```python
from build123d import *

# Parameters (mm, degrees)
F0_R        = 10
F1_DEPTH    = 25
F2_DEPTH    = 25
F3_T2_ANGLE = 203.6133668192
F3_T8_ANGLE = 184.7022290241


# Not quite as in the source:
# - a fillet or chamfer that OpenCascade refuses, or shapes differently, is made with other operations: its cross-section is extruded or revolved along the edge and cut away or added


with BuildPart() as f1:
    # F0 (on Front) → F1 (new body)
    with BuildSketch(Plane.XZ):
        with BuildLine():
            Line((4.1054428346, 24.6606029758), (0, 25))
            ThreePointArc((0, 25), (-25, 0), (0, -25))
            Line((0, -25), (4.1054428346, -24.6606029758))
            ThreePointArc((4.1054428346, -24.6606029758), (19.0740146648, -16.1611251022), (25, 0))
            ThreePointArc((25, 0), (19.0740146648, 16.1611251022), (4.1054428346, 24.6606029758))
        make_face()
        Circle(F0_R, mode=Mode.SUBTRACT)
        with BuildLine():
            ThreePointArc((4.1054428346, 24.6606029758), (2.0597239626, 24.9150062653), (0, 25))
            Line((0, 25), (4.1054428346, 24.6606029758))
        make_face()
        with BuildLine():
            Line((4.1054428346, -24.6606029758), (0, -25))
            ThreePointArc((0, -25), (2.0597239626, -24.9150062653), (4.1054428346, -24.6606029758))
        make_face()
        with BuildLine():
            Line((91.4418067738, 17.4405043857), (4.1054428346, 24.6606029758))
            ThreePointArc((4.1054428346, 24.6606029758), (19.0740146648, 16.1611251022), (25, 0))
            ThreePointArc((25, 0), (19.0740146648, -16.1611251022), (4.1054428346, -24.6606029758))
            Line((4.1054428346, -24.6606029758), (91.4418067738, -17.4405043857))
            ThreePointArc((91.4418067738, -17.4405043857), (72.5, 0), (91.4418067738, 17.4405043857))
        make_face()
        with BuildLine():
            ThreePointArc((107.5, 0), (102.8740362463, 11.8536572723), (91.4418067738, 17.4405043857))
            ThreePointArc((91.4418067738, 17.4405043857), (72.5, 0), (91.4418067738, -17.4405043857))
            ThreePointArc((91.4418067738, -17.4405043857), (102.8740362463, -11.8536572723), (107.5, 0))
        make_face()
        with Locations((90, 0)):
            Circle(F0_R, mode=Mode.SUBTRACT)
    extrude(amount=-F1_DEPTH)

    # F0 (on Front) → F2 (join)
    with BuildSketch(Plane.XZ):
        with BuildLine():
            Line((4.1054428346, 24.6606029758), (0, 25))
            ThreePointArc((0, 25), (-25, 0), (0, -25))
            Line((0, -25), (4.1054428346, -24.6606029758))
            ThreePointArc((4.1054428346, -24.6606029758), (19.0740146648, -16.1611251022), (25, 0))
            ThreePointArc((25, 0), (19.0740146648, 16.1611251022), (4.1054428346, 24.6606029758))
        make_face()
        Circle(F0_R, mode=Mode.SUBTRACT)
    extrude(amount=F2_DEPTH)

    # F3: chamfer of 2 on 4 edges, made by hand

    # F3_s1 → F3_t2 (revolve, cut)
    with BuildSketch(Plane(origin=(0, 0, 0), x_dir=(0, 1, 0), z_dir=(0.9788435281, 0, -0.2046102329))):
        Polygon((-23, 25), (-25, 23), (-25, 25), align=None)
    revolve(axis=Axis((0, -25, 0), (0, -1, 0)), revolution_arc=F3_T2_ANGLE, mode=Mode.SUBTRACT)

    # F3_s3 → F3_t4 (revolve, cut)
    with BuildSketch(Plane.XY):
        Polygon((102, 0), (100, 2), (100, 0), align=None)
    revolve(axis=Axis((90, 0, 0), (0, -1, 0)), mode=Mode.SUBTRACT)

    # F3_s5 → F3_t6 (revolve, cut)
    with BuildSketch(Plane.XY):
        Polygon((12, -25), (10, -23), (10, -25), align=None)
    revolve(axis=Axis((0, -25, 0), (0, -1, 0)), mode=Mode.SUBTRACT)

    # F3_s7 → F3_t8 (revolve, cut)
    with BuildSketch(Plane(origin=(0, 0, 0), x_dir=(0, 1, 0), z_dir=(-0.9991581953, 0, -0.0410231743))):
        Polygon((-23, -25), (-25, -23), (-25, -25), align=None)
    revolve(axis=Axis((0, -25, 0), (0, 1, 0)), revolution_arc=F3_T8_ANGLE, mode=Mode.SUBTRACT)


solid = f1.part
```
Input: part model. Units: mm. Frame: model coordinates. Round coordinates to 2 decimals unless told otherwise and drop trailing zeros. Write each loop counter-clockwise with the first axis right and the second up, starting at its lowest first coordinate (ties: lowest second). Pieces come first, ordered by that corner, then holes. Notation, with made-up numbers: M 82.25,79.25 L 101.25,79.25 A29 cw 101.25,107.25 Z; hole C 35.5,82 d2. An arc over 180 degrees is marked long. Write each question's results on one line, items separated by ' | '.
Q1. Line query: line 1 along X through (y, z) = (-23, 0.5) (1 decimal); line 2 along X through (y, z) = (9.5, 8). Output: solid intervals per line, ascending.
Results:
line 1: x = -25 to -10, 10 to 25 | line 2: x = -23.69 to -6, 6 to 84, 96 to 105.56
Q2. Section query C-C (z = -5). State how many separate pieces and enclosed holes the cut face has, and give its area (3 significant figures).
Results:
separate pieces: 3 | enclosed holes: 0 | area: 3,190 mm^2
Q3. Section query B-B (x = 90). Return loops of the section in (y, z), and give its area (3 significant figures).
Results:
outline: M 0,-17.56 L 25,-17.56 L 25,-10 L 2,-10 L 0,-12 Z; M 0,12 L 2,10 L 25,10 L 25,17.56 L 0,17.56 Z | area: 374 mm^2
Q4. Draft query along Z for faces 1 (the face through (107.496, 12.325, -0.365)), 2 (the face through (2.024, -11.381, -24.833)), 3 (the face through (80, 13, 0)). Return one class per face: released by +Z, released by -Z, zero draft, split by the parting line, or undercut.
Results:
face 1: split by the parting line | face 2: released by -Z | face 3: undercut
Q5. Section query D-D (x = 42.5). Return loops of the section in (y, z), and give its area (3 significant figures).
Results:
outline: M 0,-21.49 L 25,-21.49 L 25,21.49 L 0,21.49 Z | area: 1,070 mm^2
Q6. Section query A-A (y = 14). Return loops of the section in (x, z), and give its area (3 significant figures).
Results:
outline: M 4.11,-24.66 L 91.44,-17.44 A17.5 ccw 91.44,17.44 L 4.11,24.66 A25 ccw long Z; hole C 0,0 d20; hole C 90,0 d20 | area: 4,670 mm^2
Q7. Pin query (flat end, axial travel): P1, Ø12, axis at x = 81.5, y = 11, coming from the +Z side; P2, Ø2, axis at x = 50.5, z = 7.5, coming from the -Y side; P3, Ø10, axis at x = 40.5, y = 8, coming from the -Z side. Return the tip coordinate at first contact, or that it passes through.
Results:
P1: stops at z = 18.76 | P2: stops at y = 0 | P3: stops at z = -22.07
